Part print with two shaded views. Sizes in mm from the minimum x, y, z corner. A direction names the side the tool comes from. Coordinates: 2 decimals unless noted, no trailing zeros. Loops run counter-clockwise (first coordinate to the right, second up) from the corner with the lowest first, then second, coordinate; pieces in that order, holes last. Notation, with made-up numbers: (-12.75, 16.5) -> (20.25, 16.5) arc R20 ccw to (20.25, 41.5) -> close; hole circle Ø10 at (3.5, 38.25). An arc over 180 degrees is marked (long way). Write each question's results on one line, items separated by ' | '.
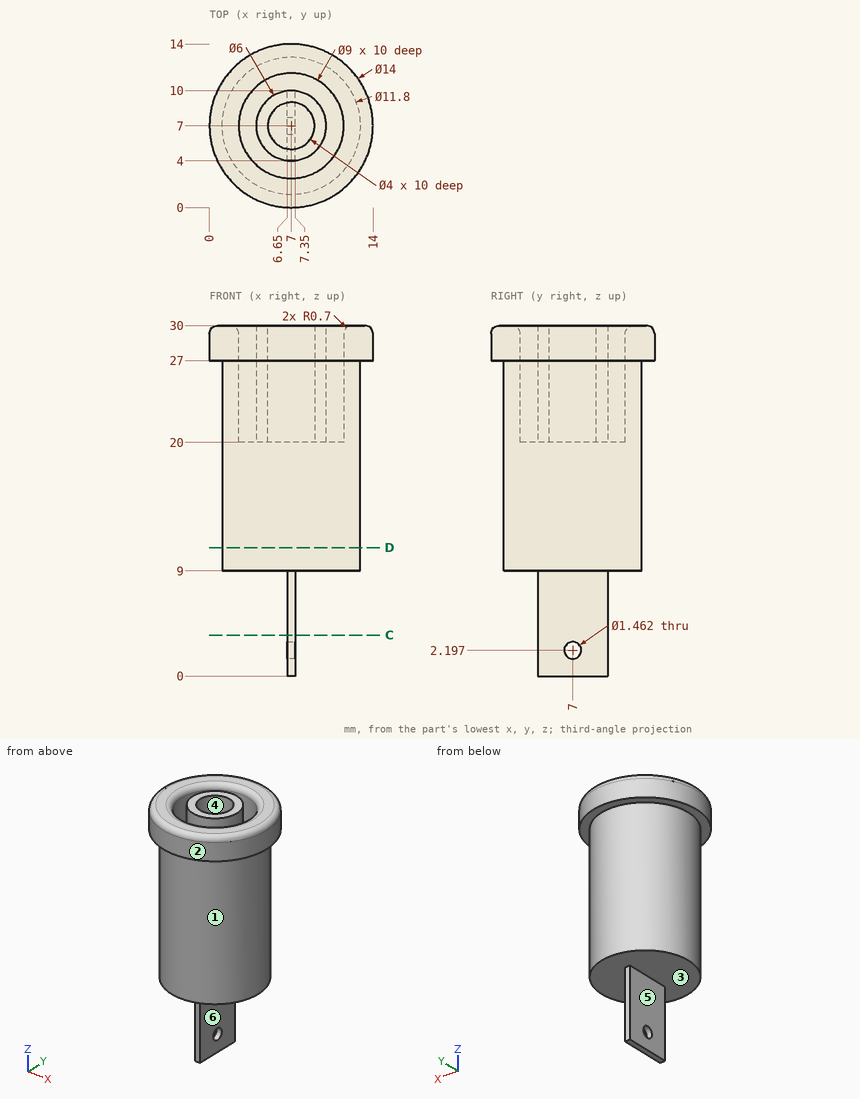
Q1. Pull direction X, two halves, no side cores. Call the marked faces 3, 4, 5 and 6: +X half, -X half, draft (parallel to the pull), parting line (faces both ways), or undercut.
Results are:
face 3: draft | face 4: undercut | face 5: -X half | face 6: +X half
Q2. Cut at D-D on z = 11. Write the cut outline in (x, y), and give its area (3 significant figures).
Results are:
outline: circle Ø11.8 at (7, 7) | area: 109 mm^2
Q3. Drop flat-ended pins along their axis: pin 1 (6 mm diameter, centred on x = 11, z = 17, fed in from +Y) (1 decimal); pin 2 (5 mm diameter, centred on y = 8.5, z = 5, fed in from +X); pin 3 (2 mm diameter, centred on x = 4.5, y = 2, fed in from -Z). Give the stop position or say it passes through.
Results are:
pin 1: y = 12.8 | pin 2: x = 7.35 | pin 3: z = 9
Q4. Which spindle directions (+Z, -Z, +X, -X, +Y, -Y) get a long thin tool onto all of the face, cutting with end or side? Do the marked faces 1 and 2. Say none if no direction does.
Results are:
face 1: -Z | face 2: +Z, -Z
Q5. Wall check: L1, parallel to Y at x = 7, z = 23; L2, parallel to Y at x = 7, z = 27.5; L3, parallel to Y at x = 9.75, z = 25.75. Give the ranges that are in metal, low to high. Write a range as from..to.
Results are:
L1: 1.1..2.5, 4..5, 9..10, 11.5..12.9 | L2: 0..2.5, 4..5, 9..10, 11.5..14 | L3: 1.78..3.44, 5.8..8.2, 10.56..12.22
Q6. Cut at C-C on z = 3.5. Write the cut outline in (x, y).
Results are:
outline: (6.65, 4) -> (7.35, 4) -> (7.35, 10) -> (6.65, 10) -> close
